Can you work these out from the model? Positions are in its coordinate system, mm. Face numbers are marked on the shaded views. A direction names the side the tool comes from. Give positions to 0.01 mm unless a question says otherwise; leave off trailing zeros. Order: outer loops, then holes, each group sorted by start corner. A loop starts at its lowest first (then second) coordinate and runs counter-clockwise, first axis right, second up. Notation, with made-up numbers: (87.25, 31.25) - (128.25, 31.25) arc R22 ccw to (128.25, 70.25) - close; hole circle Ø7 at (72.25, 14). An arc over 180 degrees is marked (long way). Answer as a JSON object with one key per item and string values.
```python
from build123d import *

# Parameters (mm, degrees)
F1_DEPTH = 27.5
F2_R     = 5
F3_R     = 3
F5_DEPTH = 5.001
F7_DEPTH = 5.001


with BuildPart() as f1:
    # F0 (on Top) → F1 (new body, symmetric)
    with BuildSketch(Plane.XY):
        Polygon((5, 0), (0, 0), (0, -50), (50, -50), (50, -45), (5, -45), align=None)
    extrude(amount=F1_DEPTH, both=True)

    # F2
    f2_edges = [f1.edges().sort_by_distance(p)[0] for p in [
        (5, -45, 0),
    ]]
    fillet(f2_edges, radius=F2_R)

    # F3
    f3_edges = [f1.edges().sort_by_distance(p)[0] for p in [
        (5, 0, 0),
        (50, -45, 0),
    ]]
    fillet(f3_edges, radius=F3_R)

    # F4 (on face) → F5 (cut, through all)
    with BuildSketch(Plane.YZ.offset(5)):
        with BuildLine():
            ThreePointArc((-16, 15), (-20, 19), (-24, 15))
            Line((-24, 15), (-24, -15))
            ThreePointArc((-24, -15), (-20, -19), (-16, -15))
            Line((-16, -15), (-16, 15))
        make_face()
    extrude(amount=-F5_DEPTH, mode=Mode.SUBTRACT)

    # F6 (on face) → F7 (cut, through all)
    with BuildSketch(Plane(origin=(0, -45, 0), x_dir=(-1, 0, 0), z_dir=(0, 1, 0))):
        with BuildLine():
            Line((-20, 4), (-35, 4))
            ThreePointArc((-35, 4), (-39, 0), (-35, -4))
            Line((-35, -4), (-20, -4))
            ThreePointArc((-20, -4), (-16, 0), (-20, 4))
        make_face()
    extrude(amount=-F7_DEPTH, mode=Mode.SUBTRACT)


solid = f1.part
```
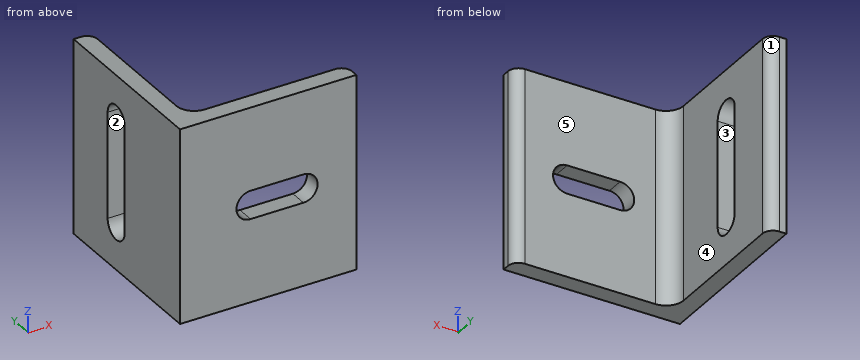
Q1. I'm going to push flat-ended pins straight in: pin 1 Ø11 at (x, z) = (37, -0.5) entering from +Y; pin 2 Ø3 at (y, z) = (-41.5, -19.5) entering from +X; pin 3 Ø10 at (y, z) = (-14.5, 6.5) entering from +X. Where does each tip first touch, or does it pass through?
Recorded:
{"pin 1": "stops at y = -45", "pin 2": "stops at x = 6", "pin 3": "stops at x = 5"}
Q2. If we section it at A-A, the plane x = 28: Please give me the cut outline in (y, z), then the cut area to 3 significant figures.
Recorded:
{"outline": "(-50, -27.5) - (-45, -27.5) - (-45, -4) - (-50, -4) - close; (-50, 4) - (-45, 4) - (-45, 27.5) - (-50, 27.5) - close", "area": "235 mm^2"}
Q3. We'd pull the mould along Y, two halves only. Please class the marked faces 3, 4 and 5: released by +Y, released by -Y, zero draft, split by the parting line, or undercut.
Recorded:
{"face 3": "undercut", "face 4": "zero draft", "face 5": "released by +Y"}
Q4. If we section it at D-D, the plane z = -6: Please give me the cut outline in (x, y).
Recorded:
{"outline": "(0, -50) - (50, -50) - (50, -48) arc R3 ccw to (47, -45) - (10, -45) arc R5 cw to (5, -40) - (5, -24) - (0, -24) - close; (0, -16) - (5, -16) - (5, -3) arc R3 ccw to (2, 0) - (0, 0) - close"}
Q5. Which directions (+Z, -Z, +X, -X, +Y, -Y) give clear straight access to the entire face, cutting with the end or side of a thin tool? Please do the marked faces 1 and 2.
Recorded:
{"face 1": "+Z, -Z, +X, +Y", "face 2": "+X, -X"}
Q6. If we section it at C-C, the plane y = -20: Please give me the cut outline in (x, z), then the cut area to 3 significant figures.
Recorded:
{"outline": "(0, -27.5) - (5, -27.5) - (5, -19) - (0, -19) - close; (0, 19) - (5, 19) - (5, 27.5) - (0, 27.5) - close", "area": "85.0 mm^2"}
Q7. I need wall thicknesses on L1, parallel to Z at x = 25, y = -47; L2, parallel to Y at x = 16.5, z = -25; L3, parallel to Y at x = 4.5, z = 18. Which ranges of each line are inside material? Lowest first, please.
Recorded:
{"L1": "z = -27.5 to -4, 4 to 27.5", "L2": "y = -50 to -45", "L3": "y = -50 to -22.65, -17.35 to -1.34"}
Q8. If we section it at B-B, the plane z = 0: Please give me the cut outline in (x, y).
Recorded:
{"outline": "(0, -50) - (16, -50) - (16, -45) - (10, -45) arc R5 cw to (5, -40) - (5, -24) - (0, -24) - close; (0, -16) - (5, -16) - (5, -3) arc R3 ccw to (2, 0) - (0, 0) - close; (39, -50) - (50, -50) - (50, -48) arc R3 ccw to (47, -45) - (39, -45) - close"}
